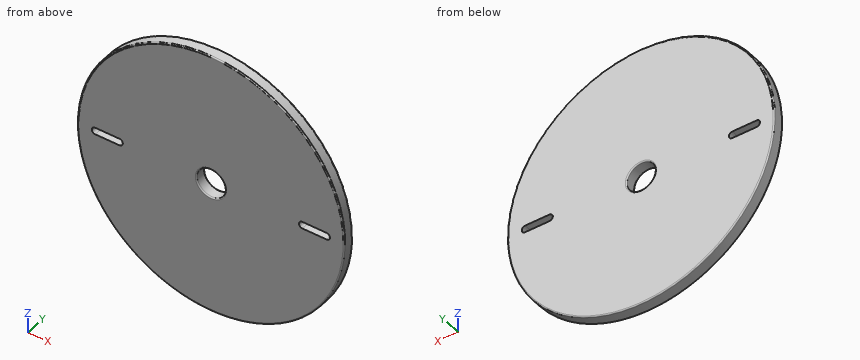
from build123d import *

# Parameters (mm, degrees)
SKETCH1_R           = 11.6
BOSS_EXTRUDE1_DEPTH = 0.5
CUT_EXTRUDE1_REACH  = 18.435
CUT_EXTRUDE2_REACH  = 18.435
SKETCH3_R           = 1.25
FILLET1_R           = 0.1


with BuildPart() as part:
    # Sketch1 → Boss-Extrude1 (new, symmetric)
    with BuildSketch(Plane(origin=(0, 0, 0), x_dir=(1, 0, 0), z_dir=(0, 1, 0))):
        with Locations(Location((0, 0, 0), (0, 0, 270))):
            Circle(SKETCH1_R)
    extrude(amount=BOSS_EXTRUDE1_DEPTH, both=True)

    # Sketch2 → Cut-Extrude1 (cut, up to next)
    with BuildSketch(Plane(origin=(0, 0.5, 0), x_dir=(1, 0, 0), z_dir=(0, 1, 0)), mode=Mode.PRIVATE) as cut_extrude1_sk1:
        with BuildLine():
            Line((-10.05, 0.3), (-7.95, 0.3))
            ThreePointArc((-7.95, 0.3), (-7.65, 0), (-7.95, -0.3))
            Line((-7.95, -0.3), (-10.05, -0.3))
            ThreePointArc((-10.05, -0.3), (-10.35, 0), (-10.05, 0.3))
        make_face()
    cut_extrude1_tool1 = extrude(cut_extrude1_sk1.sketch, amount=-CUT_EXTRUDE1_REACH, mode=Mode.PRIVATE) & part.part
    cut_extrude1 = cut_extrude1_tool1.solids().sort_by_distance((-9, 0.5, 0))[0]
    add(cut_extrude1, mode=Mode.SUBTRACT)

    # Mirror1: Cut-Extrude1 across plane
    add(cut_extrude1.mirror(Plane(origin=(0, 0, 0), x_dir=(0, 0, 1), z_dir=(1, 0, 0))), mode=Mode.SUBTRACT)

    # Sketch3 → Cut-Extrude2 (cut, up to next)
    with BuildSketch(Plane(origin=(0, 0.5, 0), x_dir=(1, 0, 0), z_dir=(0, 1, 0)), mode=Mode.PRIVATE) as cut_extrude2_sk1:
        with Locations(Location((0, 0, 0), (0, 0, 270))):
            Circle(SKETCH3_R)
    cut_extrude2_tool1 = extrude(cut_extrude2_sk1.sketch, amount=-CUT_EXTRUDE2_REACH, mode=Mode.PRIVATE) & part.part
    add(cut_extrude2_tool1.solids().sort_by_distance((0, 0.5, 0))[0], mode=Mode.SUBTRACT)

    # Fillet1
    fillet1_edges = [part.edges().sort_by_distance(p)[0] for p in [
        (0, -0.5, -11.6),
        (0, 0.5, -1.25),
        (0, -0.5, -1.25),
        (0, 0.5, -11.6),
    ]]
    fillet(fillet1_edges, radius=FILLET1_R)


solid = part.part
Can you work these out from the model? Positions are in its coordinate system, mm. Round coordinates to 2 decimals unless told otherwise and drop trailing zeros. Write each loop counter-clockwise with the first axis right and the second up, starting at its lowest first coordinate (ties: lowest second). Pieces come first, ordered by that corner, then holes. Notation, with made-up numbers: (-37, 23.25) - (-27, 23.25) arc R10 cw to (-27, 41.25) - close; hole circle Ø8 at (51, 64). An arc over 180 degrees is marked (long way). Write each question's results on one line, items separated by ' | '. Start each with the question number.
1) Suppose I cut it at C-C (z = 0). List the corners of the cut face in (x, y) for me.
2) Suppose I cut it at B-B (y = -0.1). List the corners of the cut face in (x, z) for me, and give its area (3 significant figures).
3) For pin 1 Ø0.5 at (x, y) = (-9, 0) entering from +Z; pin 2 Ø2 at (x, z) = (0, 0) entering from +Y, each with a flat end and sliding along its axis, tell me the tip position at first contact or that it passes through.
4) Please list where these lines run through material, in increasing order: line 1 (X direction, y = 0.15, z = 0); line 2 (X direction, y = 0.3, z = 1); line 3 (Z direction, x = -8, y = 0.25).
5) Suppose I cut it at A-A (x = 0). List the corners of the cut face in (y, z) for me.
Here are the results:
1) outline: (-11.6, -0.4) arc R0.1 ccw to (-11.5, -0.5) - (-10.35, -0.5) - (-10.35, 0.5) - (-11.5, 0.5) arc R0.1 ccw to (-11.6, 0.4) - close; (-7.65, -0.5) - (-1.35, -0.5) arc R0.1 ccw to (-1.25, -0.4) - (-1.25, 0.4) arc R0.1 ccw to (-1.35, 0.5) - (-7.65, 0.5) - close; (1.25, -0.4) arc R0.1 ccw to (1.35, -0.5) - (7.65, -0.5) - (7.65, 0.5) - (1.35, 0.5) arc R0.1 ccw to (1.25, 0.4) - close; (10.35, -0.5) - (11.5, -0.5) arc R0.1 ccw to (11.6, -0.4) - (11.6, 0.4) arc R0.1 ccw to (11.5, 0.5) - (10.35, 0.5) - close
2) outline: circle Ø23.2 at (0, 0); hole (-10.05, -0.3) - (-7.95, -0.3) arc R0.3 ccw to (-7.95, 0.3) - (-10.05, 0.3) arc R0.3 ccw to start; hole circle Ø2.5 at (0, 0); hole (7.95, -0.3) - (10.05, -0.3) arc R0.3 ccw to (10.05, 0.3) - (7.95, 0.3) arc R0.3 ccw to start | area: 415 mm2
3) pin 1: stops at z = 7.62 | pin 2: passes through
4) line 1: x = -11.6 to -10.35, -7.65 to -1.25, 1.25 to 7.65, 10.35 to 11.6 | line 2: x = -11.56 to -0.75, 0.75 to 11.56 | line 3: z = -8.4 to -0.3, 0.3 to 8.4
5) outline: (-0.5, -11.5) arc R0.1 ccw to (-0.4, -11.6) - (0.4, -11.6) arc R0.1 ccw to (0.5, -11.5) - (0.5, -1.35) arc R0.1 ccw to (0.4, -1.25) - (-0.4, -1.25) arc R0.1 ccw to (-0.5, -1.35) - close; (-0.5, 1.35) arc R0.1 ccw to (-0.4, 1.25) - (0.4, 1.25) arc R0.1 ccw to (0.5, 1.35) - (0.5, 11.5) arc R0.1 ccw to (0.4, 11.6) - (-0.4, 11.6) arc R0.1 ccw to (-0.5, 11.5) - close
